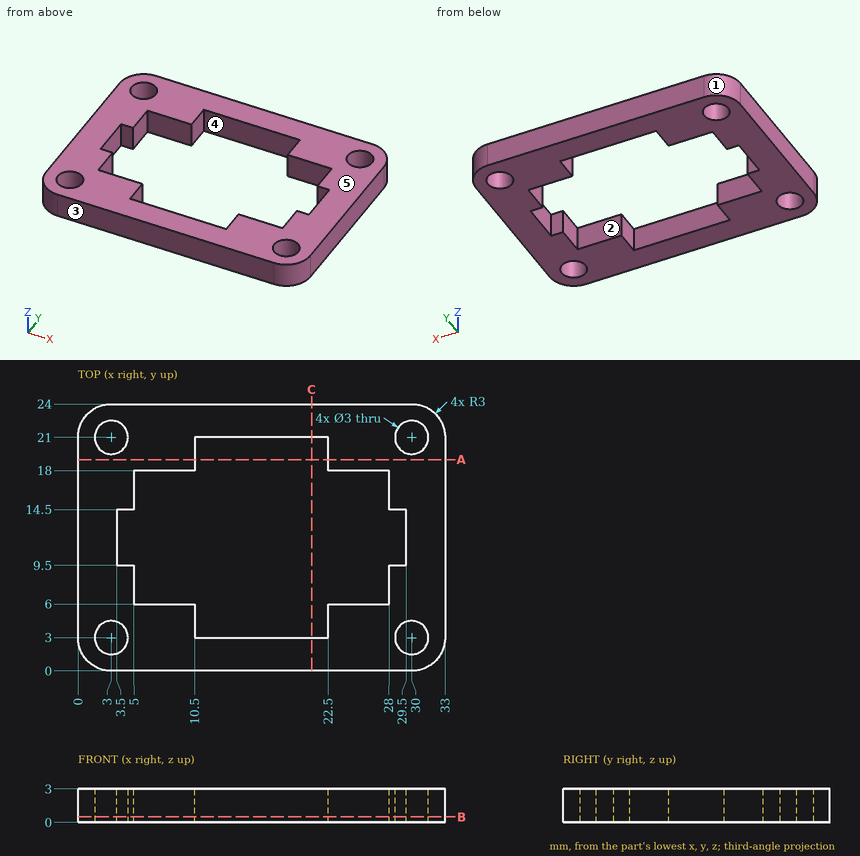
Source: three-view drawing plus pictorial views. Frame: mm from the lowest corner of the part. A direction names the side the tool comes from. Give positions to 0.01 mm unless a question says otherwise; leave off trailing zeros. Order: outer loops, then holes, each group sorted by start corner. A loop starts at its lowest first (then second) coordinate and runs counter-clockwise, first axis right, second up. Notation, with made-up numbers: (26, 10) -> (73, 10) arc R33 cw to (73, 47) -> close; hole circle Ø11 at (6.5, 44). An arc over 180 degrees is marked (long way). Put each result on its own line as item: value.
Q1. Section A-A, the plane y = 19. Return loops of the section in (x, z).
Here are the results:
outline: (0, 0) -> (10.5, 0) -> (10.5, 3) -> (0, 3) -> close; (22.5, 0) -> (33, 0) -> (33, 3) -> (22.5, 3) -> close
Q2. Draft query along Y for the marked faces 1, 2 and 3. Return one class per face: released by +Y, released by -Y, zero draft, split by the parting line, or undercut.
Here are the results:
face 1: released by +Y
face 2: undercut
face 3: released by -Y
Q3. Pin query (flat end, axial travel): pin 1 (1.2 mm diameter, centred on x = 28.5, z = 1.5, fed in from -Y). Return the tip coordinate at first contact, or that it passes through.
Here are the results:
pin 1: stops at y = 0
Q4. Section B-B, the plane z = 0.5. Count the separate pieces of the cut face and the enclosed holes in it, then the cut area to 3 significant figures.
Here are the results:
separate pieces: 1
enclosed holes: 5
area: 393 mm^2
Q5. Section C-C, the plane x = 21. Return loops of the section in (y, z).
Here are the results:
outline: (0, 0) -> (3, 0) -> (3, 3) -> (0, 3) -> close; (21, 0) -> (24, 0) -> (24, 3) -> (21, 3) -> close
Q6. Reachability of the marked faces 4 and 5 from +Z, -Z, +X, -X, +Y, -Y: full face, straight path, thin tool, end or side. Return the list, or none.
Here are the results:
face 4: +Z, -Z
face 5: +Z, +X, -X, +Y, -Y
Q7. Material intervals for L1, parallel to Y at x = 30, z = 1.05; L2, parallel to Y at x = 22, z = 1.3; L3, parallel to Y at x = 25, z = 2.5, sorted ascending.
Here are the results:
L1: y = 0 to 1.5, 4.5 to 19.5, 22.5 to 24
L2: y = 0 to 3, 21 to 24
L3: y = 0 to 6, 18 to 24
